Design review of the part built by this model. Coordinates are the model's own, in mm. Face numbers are marked on the shaded views. A direction names the side the tool comes from. Coordinates: 2 decimals unless noted, no trailing zeros. Loops run counter-clockwise (first coordinate to the right, second up) from the corner with the lowest first, then second, coordinate; pieces in that order, holes last. Notation, with made-up numbers: (83.25, -3) - (134.25, -3) arc R23 cw to (134.25, 21) - close; hole circle Ø7 at (56, -17). An arc over 180 degrees is marked (long way). Answer in a Markdown table with one row per item. Add a question column.
(1) The part is to be moulded in two halves that separate along Z. For the marked faces 3 and 4, say which applies: released by +Z, released by -Z, zero draft, split by the parting line, or undercut.
(2) To check wall thickness, follow L1, parallel to Z at x = 1, y = -17.5; L2, parallel to X at y = -2, z = -46; L3, parallel to X at y = -3.5, z = -2.5 (3 decimals). State the ranges of each line that lie inside material, in increasing order. Write a range as [from, to].
(3) Clearance check with flat-ended pins moving along their axes: pin 1 (12 mm diameter, centred on x = 69.5, y = -6.5, fed in from -Z); pin 2 (2 mm diameter, centred on x = -99, z = 75, fed in from -Y); pin 3 (1.5 mm diameter, centred on x = -90.5, y = -9.5, fed in from -Z). State where each tip first meets the part, or that it passes through.
(4) For the marked faces 1 and 2, list the 3-axis set-ups (+Z, -Z, +X, -X, +Y, -Y) from which the entire face can be reached by the end or side of a thin tool; tool diameter is ignored.
(5) We need section A-A, the plane x = -16.5. Write out the cut boundary in (y, z), plus the area to 3 significant figures.
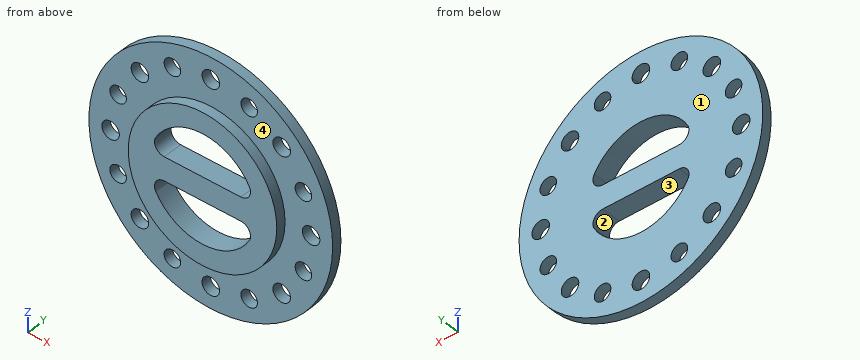
from build123d import *

# Parameters (mm, degrees)
F0_R     = 125
F0_R_2   = 9
F0_R_3   = 8.5
F0_R_4   = 76.2
F1_DEPTH = 10
F2_R     = 76.2
F3_DEPTH = 20
F5_DEPTH = 25


with BuildPart() as f1:
    # F0 (on Front) → F1 (new body)
    with BuildSketch(Plane.XZ):
        Circle(F0_R)
        with Locations((-72.7218686646, -72.6661291665)):
            Circle(F0_R_2, mode=Mode.SUBTRACT)
        with Locations((-39.3963481099, -95.0596536687)):
            Circle(F0_R_3, mode=Mode.SUBTRACT)
        with Locations((-95.0747506288, -39.3599008239)):
            Circle(F0_R_3, mode=Mode.SUBTRACT)
        with Locations((0, -102.8524214745)):
            Circle(F0_R_2, mode=Mode.SUBTRACT)
        with Locations((0, -102.8048467248)):
            Circle(F0_R_2, mode=Mode.SUBTRACT)
        with Locations((39.3599008239, -95.0747506288)):
            Circle(F0_R_3, mode=Mode.SUBTRACT)
        with Locations((72.733418035, -72.6940118133)):
            Circle(F0_R_2, mode=Mode.SUBTRACT)
        with Locations((95.0596536687, -39.3963481099)):
            Circle(F0_R_3, mode=Mode.SUBTRACT)
        with Locations((-102.8327035761, 0.0672888685)):
            Circle(F0_R_2, mode=Mode.SUBTRACT)
        with Locations((-95.0596536687, 39.3963481099)):
            Circle(F0_R_3, mode=Mode.SUBTRACT)
        with Locations((-72.6939860178, 72.7891575331)):
            Circle(F0_R_2, mode=Mode.SUBTRACT)
        with Locations((-39.3599008239, 95.0747506288)):
            Circle(F0_R_3, mode=Mode.SUBTRACT)
        Circle(F0_R_4, mode=Mode.SUBTRACT)
        with Locations((102.8721355934, 0.0278568513)):
            Circle(F0_R_2, mode=Mode.SUBTRACT)
        with Locations((95.0747506288, 39.3599008239)):
            Circle(F0_R_3, mode=Mode.SUBTRACT)
        with BuildLine():
            ThreePointArc((9.0394320172, 102.8999924447), (9.0372413226, 102.7014283411), (9.0306703054, 102.5029609028))
            ThreePointArc((9.0306703054, 102.5029609028), (-8.9583772882, 103.0985565482), (9.0394320172, 102.8999924447))
        make_face(mode=Mode.SUBTRACT)
        with BuildLine():
            ThreePointArc((47.8963481099, 95.0596536687), (47.6968165425, 93.2287457523), (47.1075895691, 91.4837964067))
            ThreePointArc((47.1075895691, 91.4837964067), (36.1420336402, 87.2073013248), (31.4162857275, 97.9868715241))
            ThreePointArc((31.4162857275, 97.9868715241), (40.8828658107, 103.4286598895), (47.8963481099, 95.0596536687))
        make_face(mode=Mode.SUBTRACT)
        with BuildLine():
            ThreePointArc((66.1251217448, 78.84084141), (76.0227719424, 81.1495288892), (81.7613006818, 72.7612748864))
            ThreePointArc((81.7613006818, 72.7612748864), (69.4998294213, 64.3730208835), (66.1251217448, 78.84084141))
        make_face(mode=Mode.SUBTRACT)
    extrude(amount=F1_DEPTH)

    # F2 (on Front) → F3 (join)
    with BuildSketch(Plane.XZ):
        Circle(F2_R)
    extrude(amount=F3_DEPTH)

    # F4 (on face) → F5 (cut)
    with BuildSketch(Plane.XZ.offset(20)):
        with BuildLine():
            ThreePointArc((-47.9790334867, 26.8888888889), (-47.8836922565, 16.944749704), (-39.2555728528, 12))
            Line((-39.2555728528, 12), (39.2555728528, 12))
            ThreePointArc((39.2555728528, 12), (47.8836922565, 16.944749704), (47.9790334867, 26.8888888889))
            ThreePointArc((47.9790334867, 26.8888888889), (0, 55), (-47.9790334867, 26.8888888889))
        make_face()
        with BuildLine():
            ThreePointArc((-39.2555728528, -12), (-47.8836922565, -16.944749704), (-47.9790334867, -26.8888888889))
            ThreePointArc((-47.9790334867, -26.8888888889), (0, -55), (47.9790334867, -26.8888888889))
            ThreePointArc((47.9790334867, -26.8888888889), (47.8836922565, -16.944749704), (39.2555728528, -12))
            Line((39.2555728528, -12), (-39.2555728528, -12))
        make_face()
    extrude(amount=-F5_DEPTH, mode=Mode.SUBTRACT)


solid = f1.part
Responses:
| question | item | result |
|---|---|---|
| 1 | face 3 | undercut |
| 1 | face 4 | zero draft |
| 2 | L1 | z = [-76.19, -54.99], [-12, 12], [54.99, 76.19] |
| 2 | L2 | x = [-116.23, -100.38], [-89.77, -30.15], [30.15, 89.71], [100.41, 116.23] |
| 2 | L3 | x = [-124.975, -111.459], [-94.207, 94.234], [111.51, 124.975] |
| 3 | pin 1 | stops at z = -107.67 |
| 3 | pin 2 | stops at y = -10 |
| 3 | pin 3 | stops at z = -87.01 |
| 4 | face 1 | +Z, -Z, +X, -X, +Y |
| 4 | face 2 | +Y, -Y |
| 5 | outline | (-20, -74.39) - (-10, -74.39) - (-10, -123.91) - (0, -123.91) - (0, -52.47) - (-20, -52.47) - close; (-20, -12) - (0, -12) - (0, 12) - (-20, 12) - close; (-20, 52.47) - (0, 52.47) - (0, 123.91) - (-10, 123.91) - (-10, 74.39) - (-20, 74.39) - close |
| 5 | area | 2,350 mm2 |
